Can you work these out from the model? Positions are in its coordinate system, mm. Give positions to 0.01 mm unless a question says otherwise; leave off trailing zeros. Loops run counter-clockwise (first coordinate to the right, second up) from the corner with the lowest first, then second, coordinate; pieces in that order, holes last. Notation, with made-up numbers: (70.5, -37) -> (122.5, -37) arc R18 cw to (122.5, -20) -> close; hole circle Ø6 at (-12.75, 15.25). An arc over 180 degrees is marked (long way). Return JSON: item names as keys, results as strings. Group by question number.
Q1. I need wall thicknesses on line 1 along Z through (x, y) = (17.5, -1.55); line 2 along Z through (x, y) = (150, -1.1). Which ranges of each line are inside material? Lowest first, please. Write a range as [from, to].
Q2. Suppose I cut it at B-B, the plane x = 17.5. Please give me the cut outline in (y, z), and give its area (3 significant figures).
Q3. Thinking about a two-plate mould opening in X: for faces 1 (the flat face through (-2, -2, 1)), 2 (the cylindrical face through (-18.021, -1.014, -36.034)), which applies, pulls with the +X half, pulls with the -X half, needs draft (parallel to the pull), parting line crosses it, or undercut?
Q4. Suppose I cut it at A-A, the plane z = -40. Please give me the cut outline in (x, y), and give its area (3 significant figures).
```python
from build123d import *

# Parameters (mm, degrees)
F0_W     = 350
F0_H     = 150
F1_DEPTH = 2
F2_R     = 4
F3_DEPTH = 25
F5_D     = 5.5
F5_DEPTH = 13
F5_TIP   = 1.6523667023


with BuildPart() as f1:
    # F0 (on Front) → F1 (new body)
    with BuildSketch(Plane.XZ):
        Rectangle(F0_W, F0_H)
    extrude(amount=F1_DEPTH)

    # F2 (on face) → F3 (cut)
    with BuildSketch(Plane.XZ.offset(2)):
        with Locations((-17.5, -40)):
            Circle(F2_R)
        with Locations((17.5, -40)):
            Circle(F2_R)
    extrude(amount=-F3_DEPTH, mode=Mode.SUBTRACT)

    # F5
    with Locations(Plane.XZ.offset(2)):
        with Locations((-150, -70.5), (-50, -70.5), (50, -70.5), (150, -70.5)):
            Hole(F5_D / 2, depth=F5_DEPTH)
            with Locations((0, 0, -(F5_DEPTH + F5_TIP / 2))):  # 118° drill point
                Cone(0, F5_D / 2, F5_TIP, mode=Mode.SUBTRACT)


solid = f1.part
```
Ans:
{
 "1": {"line 1": "z = [-75, -44], [-36, 75]", "line 2": "z = [-75, -73.25], [-67.75, 75]"},
 "2": {"outline": "(-2, -75) -> (0, -75) -> (0, -44) -> (-2, -44) -> close; (-2, -36) -> (0, -36) -> (0, 75) -> (-2, 75) -> close", "area": "284 mm^2"},
 "3": {"face 1": "needs draft", "face 2": "undercut"},
 "4": {"outline": "(-175, -2) -> (-21.5, -2) -> (-21.5, 0) -> (-175, 0) -> close; (-13.5, -2) -> (13.5, -2) -> (13.5, 0) -> (-13.5, 0) -> close; (21.5, -2) -> (175, -2) -> (175, 0) -> (21.5, 0) -> close", "area": "668 mm^2"}
}
